Design review of the part shown in the three views and the two pictorial views. Dimensions are in mm from the part's minimum x, y and z. Round coordinates to 2 decimals unless told otherwise and drop trailing zeros. Loops run counter-clockwise (first coordinate to the right, second up) from the corner with the lowest first, then second, coordinate; pieces in that order, holes last.
1. Consider section A-A on y = 9.95. State the section outline as (x, z) points.
2. Draft analysis for pull direction Z (two halves, no side actions). For the marked faces 1, 2 and 3, state which applies: released by +Z, released by -Z, zero draft, split by the parting line, or undercut.
3. To check wall thickness, follow line 1 along X through (y, z) = (14, 2.5); line 2 along Y through (x, z) = (15, 2.25); line 3 along X through (y, z) = (4, 3.05). State the ranges of each line that lie inside material, in increasing order.
4. Consider section D-D on x = 15. State the section outline as (y, z) points, then the cut area to 3 significant figures.
5. Consider section B-B on z = 2.5. State the section outline as (x, y) points, then the cut area to 3 significant figures.
6. Consider section C-C on x = 7. State the section outline as (y, z) points.
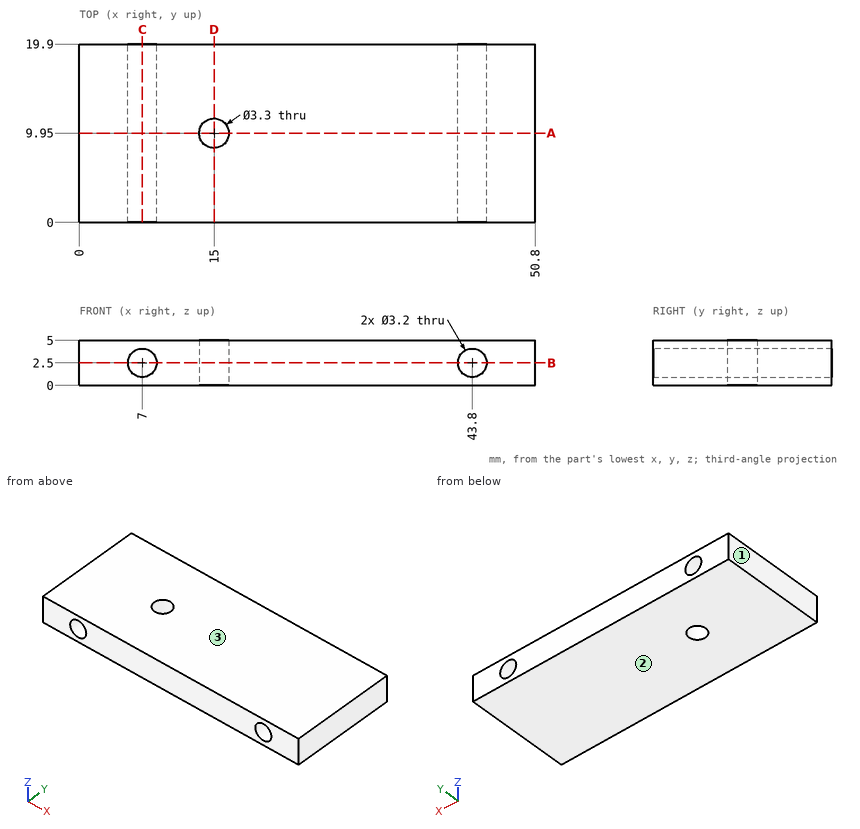
Resolved:
1. outline: (0, 0) - (13.35, 0) - (13.35, 5) - (0, 5) - close; (16.65, 0) - (50.8, 0) - (50.8, 5) - (16.65, 5) - close; hole circle Ø3.2 at (7, 2.5); hole circle Ø3.2 at (43.8, 2.5)
2. face 1: zero draft
2. face 2: released by -Z
2. face 3: released by +Z
3. line 1: x = 0 to 5.4, 8.6 to 42.2, 45.4 to 50.8
3. line 2: y = 0 to 8.3, 11.6 to 19.9
3. line 3: x = 0 to 5.5, 8.5 to 42.3, 45.3 to 50.8
4. outline: (0, 0) - (8.3, 0) - (8.3, 5) - (0, 5) - close; (11.6, 0) - (19.9, 0) - (19.9, 5) - (11.6, 5) - close
4. area: 83.0 mm2
5. outline: (0, 0) - (5.4, 0) - (5.4, 19.9) - (0, 19.9) - close; (8.6, 0) - (42.2, 0) - (42.2, 19.9) - (8.6, 19.9) - close; (45.4, 0) - (50.8, 0) - (50.8, 19.9) - (45.4, 19.9) - close; hole circle Ø3.3 at (15, 9.95)
5. area: 875 mm2
6. outline: (0, 0) - (19.9, 0) - (19.9, 0.9) - (0, 0.9) - close; (0, 4.1) - (19.9, 4.1) - (19.9, 5) - (0, 5) - close
